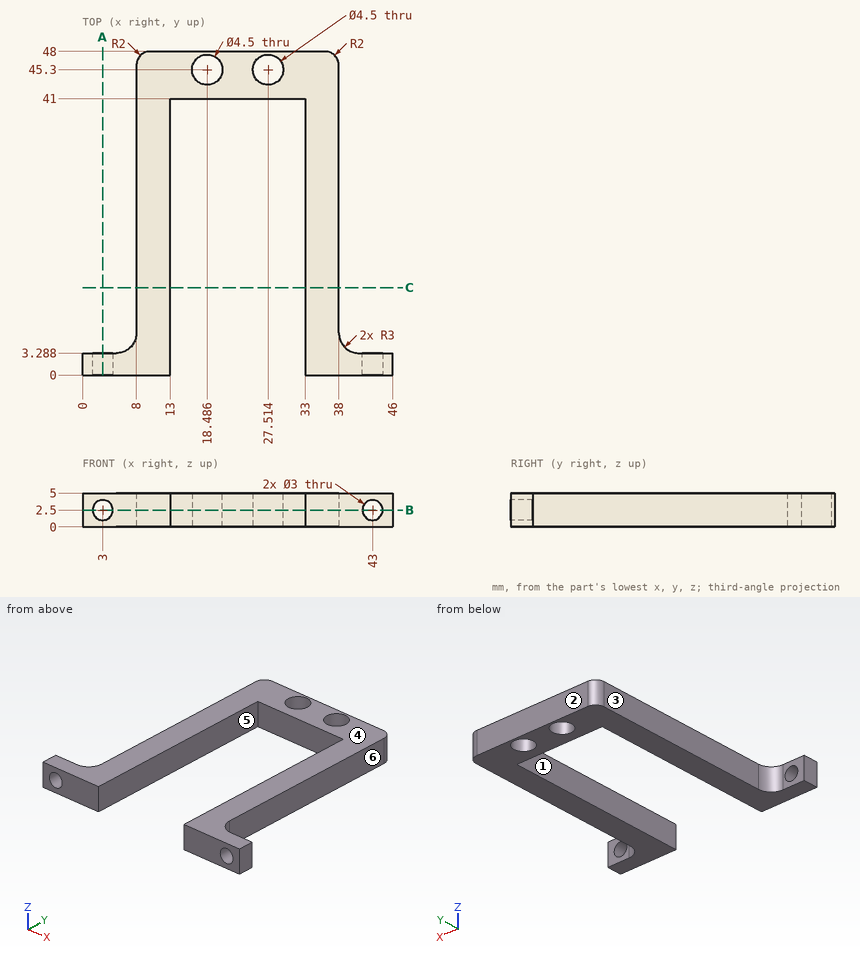
Geometry check sheet. Reference: drawing and pictorial views, mm from the part's lowest x, y, z. A direction names the side the tool comes from. Round coordinates to 2 decimals unless told otherwise and drop trailing zeros. Write each loop counter-clockwise with the first axis right and the second up, starting at its lowest first coordinate (ties: lowest second). Pieces come first, ordered by that corner, then holes.
1. Section check B-B on z = 2.5. Enter the section's corners in (x, y), plus the area to 3 significant figures.
2. Section check C-C on y = 13. Enter the section's corners in (x, z).
3. Draft check along X on the marked faces 4, 5 and 6. Enter one of: +X half, -X half, draft (parallel to the pull), parting line (faces both ways), or undercut.
4. Access from +Z, -Z, +X, -X, +Y, -Y to the whole of each face (thin tool, end or side, straight path). Record for the marked faces 1, 2 and 3.
5. Section check A-A on x = 3. Enter the section's corners in (y, z).
6. Gauge pin test, flat ends, axial feed: P1, Ø3, axis at y = 16.5, z = 3.5, coming from the +X side; P2, Ø1.5, axis at y = 19.5, z = 2, coming from the -X side; P3, Ø1.5, axis at x = 25, z = 3.5, coming from the -Y side. Record the tip position at first contact, or that the pin passes through.
7. Scan lines: L1, parallel to X at y = 1.1, z = 2.5; L2, parallel to X at y = 45.3, z = 3.7; L3, parallel to X at y = 27.5, z = 3.5. Record each from-to range of solid material in increasing order.
Answer:
1. outline: (0, 0) - (1.5, 0) - (1.5, 3.29) - (0, 3.29) - close; (4.5, 0) - (13, 0) - (13, 41) - (33, 41) - (33, 0) - (41.5, 0) - (41.5, 3.29) - (41, 3.29) arc R3 cw to (38, 6.29) - (38, 46) arc R2 ccw to (36, 48) - (10, 48) arc R2 ccw to (8, 46) - (8, 6.29) arc R3 cw to (5, 3.29) - (4.5, 3.29) - close; (44.5, 0) - (46, 0) - (46, 3.29) - (44.5, 3.29) - close; hole circle Ø4.5 at (18.49, 45.3); hole circle Ø4.5 at (27.51, 45.3)
1. area: 623 mm2
2. outline: (8, 0) - (13, 0) - (13, 5) - (8, 5) - close; (33, 0) - (38, 0) - (38, 5) - (33, 5) - close
3. face 4: draft
3. face 5: undercut
3. face 6: +X half
4. face 1: +Z, -Z, -Y
4. face 2: +Z, -Z, +X, -X, +Y
4. face 3: +Z, -Z, -X, +Y
5. outline: (0, 0) - (3.29, 0) - (3.29, 1) - (0, 1) - close; (0, 4) - (3.29, 4) - (3.29, 5) - (0, 5) - close
6. P1: stops at x = 38
6. P2: stops at x = 8
6. P3: stops at y = 41
7. L1: x = 0 to 1.5, 4.5 to 13, 33 to 41.5, 44.5 to 46
7. L2: x = 8 to 16.24, 20.74 to 25.26, 29.76 to 38
7. L3: x = 8 to 13, 33 to 38
